Source: three-view drawing plus pictorial views. Frame: mm from the lowest corner of the part. A direction names the side the tool comes from. Coordinates: 2 decimals unless noted, no trailing zeros. Loops run counter-clockwise (first coordinate to the right, second up) from the corner with the lowest first, then second, coordinate; pieces in that order, holes last. Notation, with made-up numbers: M 20,-28 L 58,-28 A37 cw 58,8 Z; hole C -37,59.5 d5. An arc over 180 degrees is marked long. Use a Markdown table: item, result. Add a question column.
1. Section B-B on z = 30. Output: boundary loops of the cut face in (x, y), then the cut area to 3 significant figures.
2. Section A-A on z = 17.78. Output: boundary loops of the cut face in (x, y).
3. Pin query (flat end, axial travel): pin 1 (1 mm diameter, centred on x = 26.5, y = 23.5, fed in from -Z); pin 2 (7.5 mm diameter, centred on y = 19.05, z = 17.78, fed in from -X). Return the tip coordinate at first contact, or that it passes through.
4. Line query: L1, parallel to X at y = 48, z = 26; L2, parallel to Z at x = 105.5, y = 19.05. Output: solid intervals per line, ascending. Write a range as [from, to].
5. Section D-D on y = 88. Output: boundary loops of the cut face in (x, z), then the cut area to 3 significant figures.
6. Draft query along X for the marked faces 1, 2, 3 and 4. Return one class per face: +X half, -X half, draft (parallel to the pull), parting line (faces both ways), or undercut.
7. Section C-C on y = 19.05. Output: boundary loops of the cut face in (x, z), then the cut area to 3 significant figures.
8. Set-up query: the marked faces 5 and 6. Return all of +Z, -Z, +X, -X, +Y, -Y with unobstructed straight access to the full face (end or side cutting, diameter ignored); none if empty.
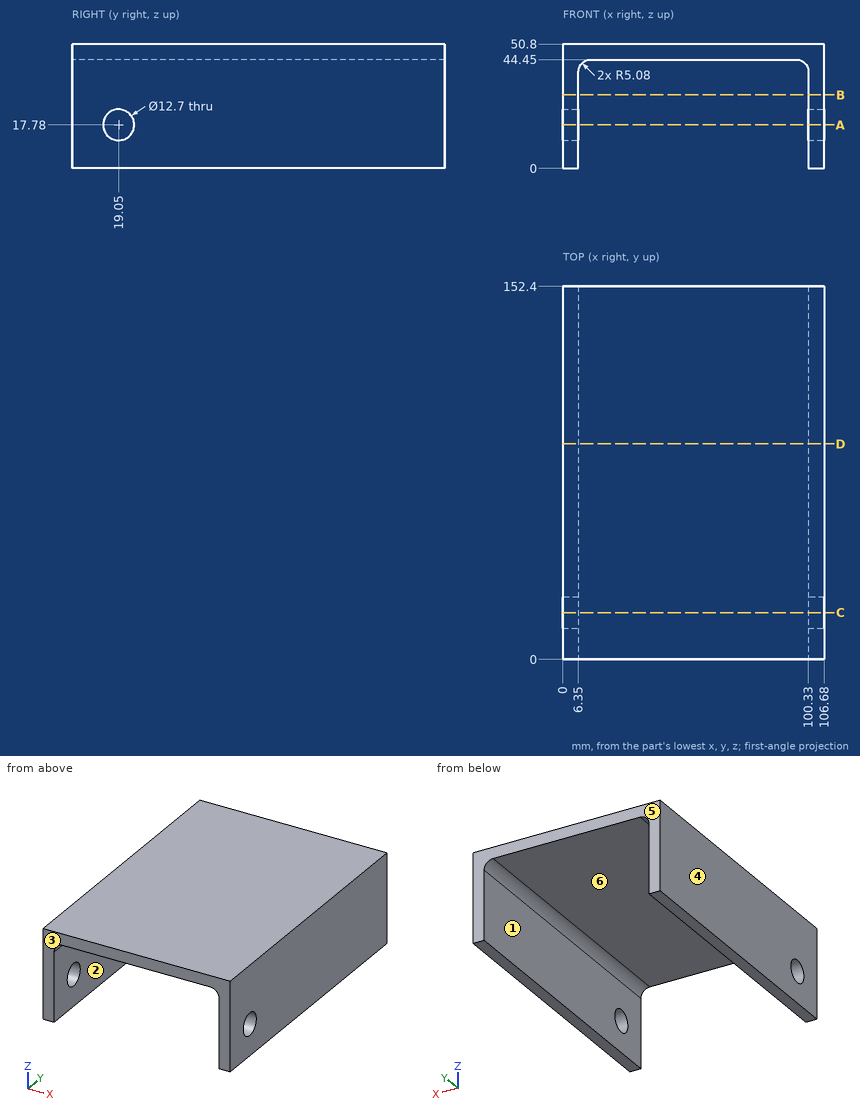
Answers below:
| question | item | result |
|---|---|---|
| 1 | outline | M 0,0 L 6.35,0 L 6.35,152.4 L 0,152.4 Z; M 100.33,0 L 106.68,0 L 106.68,152.4 L 100.33,152.4 Z |
| 1 | area | 1,940 mm² |
| 2 | outline | M 0,0 L 6.35,0 L 6.35,12.7 L 0,12.7 Z; M 0,25.4 L 6.35,25.4 L 6.35,152.4 L 0,152.4 Z; M 100.33,0 L 106.68,0 L 106.68,12.7 L 100.33,12.7 Z; M 100.33,25.4 L 106.68,25.4 L 106.68,152.4 L 100.33,152.4 Z |
| 3 | pin 1 | stops at z = 44.45 |
| 3 | pin 2 | passes through |
| 4 | L1 | x = [0, 6.35], [100.33, 106.68] |
| 4 | L2 | z = [0, 11.43], [24.13, 50.8] |
| 5 | outline | M 0,0 L 6.35,0 L 6.35,39.37 A5.08 cw 11.43,44.45 L 95.25,44.45 A5.08 cw 100.33,39.37 L 100.33,0 L 106.68,0 L 106.68,50.8 L 0,50.8 Z |
| 5 | area | 1,250 mm² |
| 6 | face 1 | undercut |
| 6 | face 2 | undercut |
| 6 | face 3 | draft |
| 6 | face 4 | -X half |
| 7 | outline | M 0,0 L 6.35,0 L 6.35,11.43 L 0,11.43 Z; M 0,24.13 L 6.35,24.13 L 6.35,39.37 A5.08 cw 11.43,44.45 L 95.25,44.45 A5.08 cw 100.33,39.37 L 100.33,24.13 L 106.68,24.13 L 106.68,50.8 L 0,50.8 Z; M 100.33,0 L 106.68,0 L 106.68,11.43 L 100.33,11.43 Z |
| 7 | area | 1,090 mm² |
| 8 | face 5 | +Z, -Z, +X, -X, +Y |
| 8 | face 6 | -Z, +Y, -Y |
